Autodesk Inventor part; units mm, degrees
ref_plane "Plano de trabajo2" through (2.75, 0, 0) normal (1, 0, 0) x (0, 1, 0)
ref_plane "Plano de trabajo3" through (-2.75, 0, 0) normal (1, 0, 0) x (0, 1, 0)
ref_plane "Plano de trabajo6" through (2.75, 0, 0) normal (1, 0, 0) x (0, 1, 0)
sketch "Boceto1" plane through (0, 0, 0) normal (0, 0, 1) x (1, 0, 0)
  arc A0 (0, -2.75) -> (0, 2.75) centre (0, 0) ccw
  line L0 (0, 2.75) -> (0, -2.75)
  dimension "d0" = 5.5
revolve "Revolución1" add sketch "Boceto1" angle 360 about axis through (0, 2.75, 0) along (0, -1, 0)
ref_plane "Plano de trabajo2" through (2.75, 0, 0) normal (1, 0, 0) x (0, 1, 0)
ref_plane "Plano de trabajo3" through (-2.75, 0, 0) normal (1, 0, 0) x (0, 1, 0)
sketch "Boceto7" plane through (2.75, 0, 0) normal (1, 0, 0) x (0, 1, 0)
  circle A0 centre (0, 0) radius 1.7
  circle A1 centre (0, 0) radius 1.3
  dimension "d21" = 3.4
  dimension "d22" = 0.4
extrude "Extrusión5" add sketch "Boceto7" along normal blind 0.5 and the other way blind 1
sketch "Boceto8" plane through (-2.75, 0, 0) normal (1, 0, 0) x (0, 1, 0)
  circle A0 centre (0, 0) radius 1.7
  circle A1 centre (0, 0) radius 1.7
  circle A2 centre (0, 0) radius 1.3
  dimension "d27" = 3.4
  dimension "d35" = 2.6
extrude "Extrusión6" add sketch "Boceto8" along normal blind 1 and the other way blind 0.5 contours A0 | A2
ref_plane "Plano de trabajo6" through (2.75, 0, 0) normal (1, 0, 0) x (0, 1, 0)
sketch "Boceto10" plane through (2.75, 0, 0) normal (1, 0, 0) x (0, 1, 0)
  circle A0 centre (0, 0) radius 1.3
extrude "Extrusión8" cut sketch "Boceto10" against normal blind 10
properties part number "Bola chica" material "Aluminio 6061"
Source: CAD feature listing. Evaluate the final solid. Frame: model axes, mm. Give positions to 0.01 mm unless a question says otherwise; leave off trailing zeros. Write each loop counter-clockwise with the first axis right and the second up, starting at its lowest first coordinate (ties: lowest second). Pieces come first, ordered by that corner, then holes. Notation, with made-up numbers: (11.25, -4) - (33.25, -4) arc R23 cw to (33.25, 32) - close; hole circle Ø11 at (87, -9). An arc over 180 degrees is marked (long way). One line per item, written item: value. Start each with the question number.
Q1. Section query A-A, the plane y = 0. Return the cut outline in (x, z), then the cut area to 3 significant figures.
Q2. Draft query along Z for faces 1 (the face through (-2.7, -0.37, -1.66)), 2 (the face through (-0.05, -0.17, -1.29)). Return one class per face: +Z half, -Z half, draft (parallel to the pull), parting line (faces both ways), or undercut.
Q3. Section query C-C, the plane z = 1.45. Return the cut outline in (x, y), then the cut area to 3 significant figures.
Q4. First-contact query: pin 1 Ø1.5 at (x, z) = (-2, 2) entering from +Y; pin 2 Ø2 at (x, y) = (-2.5, 2) entering from +Z; pin 3 Ø2 at (y, z) = (0, 0) entering from +X. Flat tips, straight axial feed; report the tip coordinate or a pass-through.
Q5. Material intervals for probe 1 along Y at (x, z) = (-0.25, -0.45); probe 2 along Z at (x, y) = (1, -0.55); probe 3 along Y at (x, z) = (1.5, 0.75), sorted ascending. Write a range as from..to.
Q6. Section query D-D, the plane x = -1. Return the cut outline in (y, z), then the cut area to 3 significant figures.
Answer:
1. outline: (-3.25, -1.7) - (-2.16, -1.7) arc R2.75 ccw to (2.16, -1.7) - (3.25, -1.7) - (3.25, -1.3) - (-3.25, -1.3) - close; (-3.25, 1.3) - (3.25, 1.3) - (3.25, 1.7) - (2.16, 1.7) arc R2.75 ccw to (-2.16, 1.7) - (-3.25, 1.7) - close
1. area: 11.5 mm2
2. face 1: parting line
2. face 2: undercut
3. outline: (-3.25, -0.89) - (-2.16, -0.89) arc R2.34 ccw to (2.16, -0.89) - (3.25, -0.89) - (3.25, 0.89) - (2.16, 0.89) arc R2.34 ccw to (-2.16, 0.89) - (-3.25, 0.89) - close
3. area: 20.6 mm2
4. pin 1: stops at y = 1.8
4. pin 2: stops at z = 1.65
4. pin 3: passes through
5. probe 1: y = -2.7..-1.22, 1.22..2.7
5. probe 2: z = -2.5..-1.18, 1.18..2.5
5. probe 3: y = -2.18..-1.06, 1.06..2.18
6. outline: circle Ø5.12 at (0, 0); hole circle Ø2.6 at (0, 0)
6. area: 15.3 mm2
